Drawing for the job (mm, zero at the part's lowest x, y, z). A direction names the side the tool comes from. Coordinates: 2 decimals unless noted, no trailing zeros. Write each loop counter-clockwise with the first axis right and the second up, starting at its lowest first coordinate (ties: lowest second). Pieces come first, ordered by that corner, then holes. Notation, with made-up numbers: M 15,-33.5 L 66,-33.5 A26 ccw 66,-15.5 Z; hole C 22.5,67 d4. An arc over 180 degrees is marked long. Put each result on its own line as item: value. Start each with the question number.
Q1. Pull direction X, two halves, no side cores. Call the marked faces 4, 5 and 6: pulls with the +X half, pulls with the -X half, needs draft (parallel to the pull), parting line crosses it, or undercut.
Q2. Drop flat-ended pins along their axis: pin 1 (2 mm diameter, centred on x = 6.5, z = 6.5, fed in from -Y); pin 2 (4 mm diameter, centred on y = 9, z = 9, fed in from -X); pin 3 (2 mm diameter, centred on y = 5.5, z = 2, fed in from +X); pin 4 (1 mm diameter, centred on x = 7.5, z = 4.5, fed in from +Y). Give the stop position or say it passes through.
Q3. Cut at B-B (x = 8.9). Write the cut outline in (y, z), then the cut area to 3 significant figures.
Q4. Cut at C-C (y = 5.5). Write the cut outline in (x, z).
Q5. Cut at D-D (z = 4.5). Write the cut outline in (x, y).
Q6. Drill centre lines: line 1 along X through (y, z) = (7.25, 6); line 2 along Y through (x, z) = (8.5, 8.25); line 3 along X through (y, z) = (12.75, 4.5). Where is each one in solid material? Low to high.
Q7. Which spindle directions (+Z, -Z, +X, -X, +Y, -Y) get a long thin tool onto all of the face, cutting with end or side? Do the marked faces 1, 2 and 3. Say none if no direction does.
Q8. Cut at A-A (y = 8). Write the cut outline in (x, z).
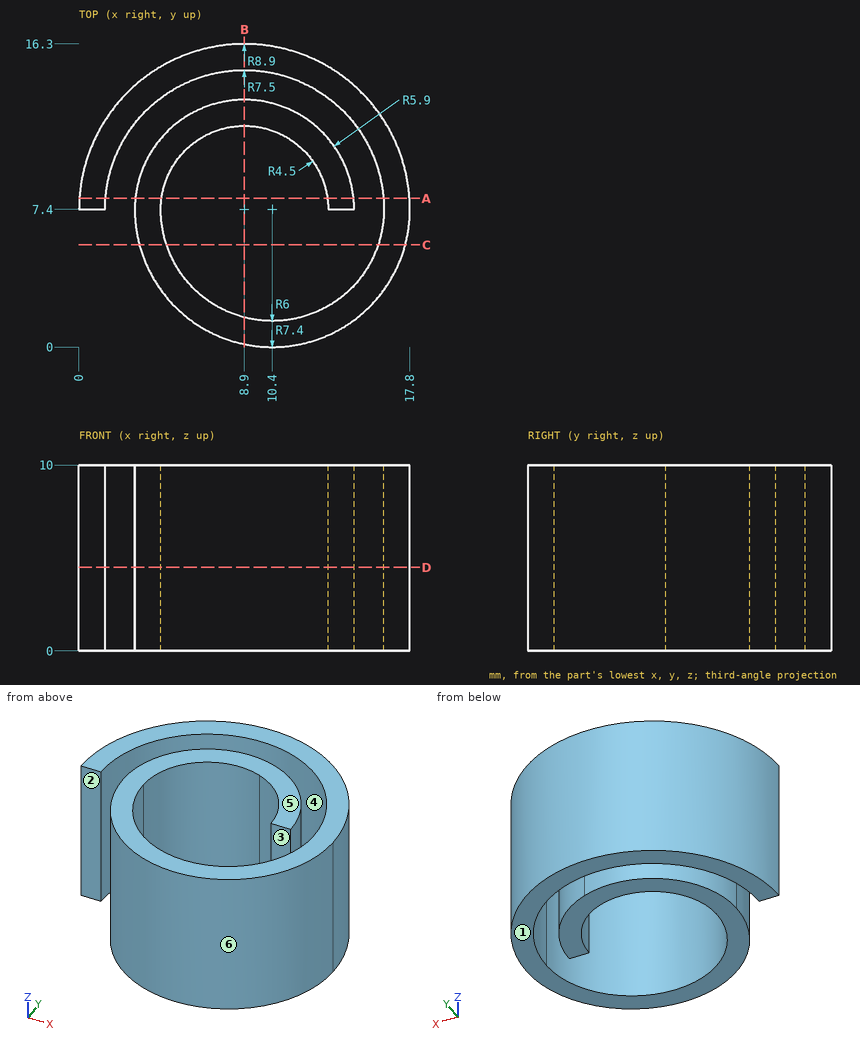
Computed values:
1. face 4: undercut
1. face 5: needs draft
1. face 6: parting line crosses it
2. pin 1: y = 0.59
2. pin 2: x = 0
2. pin 3: x = 17.75
2. pin 4: y = 16.25
3. outline: M 0.15,0 L 1.59,0 L 1.59,10 L 0.15,10 Z; M 11.9,0 L 13.3,0 L 13.3,10 L 11.9,10 Z; M 14.9,0 L 16.3,0 L 16.3,10 L 14.9,10 Z
3. area: 42.4 mm2
4. outline: M 3.25,0 L 4.71,0 L 4.71,10 L 3.25,10 Z; M 16.09,0 L 17.55,0 L 17.55,10 L 16.09,10 Z
5. outline: M 0,7.4 L 1.4,7.4 A7.5 cw 16.4,7.4 A6 cw 4.4,7.4 A4.5 cw 13.4,7.4 L 14.8,7.4 A5.9 ccw 10.87,12.96 A5.9 ccw 3,7.4 A7.4 ccw 17.8,7.4 A8.9 ccw Z
6. line 1: 3 to 4.4, 16.4 to 17.8
6. line 2: 0.25 to 1.71, 11.88 to 13.29, 14.89 to 16.29
6. line 3: 1.79 to 3.64, 6.41 to 11.39, 14.16 to 16.01
7. face 1: -Z, +X, -X, +Y, -Y
7. face 2: +Z, -Z, -X, -Y
7. face 3: +Z, -Z
8. outline: M 0.02,0 L 1.42,0 L 1.42,10 L 0.02,10 Z; M 3.03,0 L 4.44,0 L 4.44,10 L 3.03,10 Z; M 13.36,0 L 14.77,0 L 14.77,10 L 13.36,10 Z; M 16.38,0 L 17.78,0 L 17.78,10 L 16.38,10 Z
